```python
from build123d import *

# Parameters (mm, degrees)
SKETCH1_W                    = 40
SKETCH1_H                    = 55
BOSS_EXTRUDE1_DEPTH          = 2
CONVERT_SOLID1_START         = -20
CONVERT_SOLID1_OUTLINE_W     = 55
CONVERT_SOLID1_OUTLINE_H     = 1
CONVERT_SOLID1_DEPTH         = 40
EDGE_FLANGE1_STRIP_W         = 18
EDGE_FLANGE1_STRIP_H         = 3
EDGE_FLANGE1_STRIP_CUT_DEPTH = 40
EDGE_FLANGE1_DEPTH           = 40
SKETCH10_R                   = 2.25
CUT_EXTRUDE1_DEPTH           = 58.965506985


# Read off the part's stored shape, not the designer's step: Convert-Solid1
# Sheet-metal steps are written as plain solids
with BuildPart() as part:
    # Sketch1 → Boss-Extrude1 (new body)
    with BuildSketch(Plane.XY):
        Rectangle(SKETCH1_W, SKETCH1_H)
    extrude(amount=BOSS_EXTRUDE1_DEPTH)

    # Convert-Solid1 outline → Convert-Solid1 (add)
    with BuildSketch(Plane.YZ.offset(CONVERT_SOLID1_START)):
        with Locations((0, -0.5)):
            Rectangle(CONVERT_SOLID1_OUTLINE_W, CONVERT_SOLID1_OUTLINE_H)
    extrude(amount=CONVERT_SOLID1_DEPTH)

    # Edge-Flange1 strip (across the edge) → Edge-Flange1 strip cut (cut)
    with BuildSketch(Plane(origin=(-20, 27.5, -1), x_dir=(0, -1, 0), z_dir=(1, 0, 0))):
        with Locations((-3, -1.5)):
            Rectangle(EDGE_FLANGE1_STRIP_W, EDGE_FLANGE1_STRIP_H)
    extrude(amount=EDGE_FLANGE1_STRIP_CUT_DEPTH, mode=Mode.SUBTRACT)

    # Edge-Flange1 section (across the edge) → Edge-Flange1 (add)
    with BuildSketch(Plane(origin=(-20, 27.5, -1), x_dir=(0, -1, 0), z_dir=(1, 0, 0))):
        with BuildLine():
            Line((0, 3), (0, 15))
            Line((0, 15), (3, 15))
            Line((3, 15), (3, 3))
            ThreePointArc((3, 3), (3.878679656, 0.878679656), (6, 0))
            Line((6, 0), (6, -3))
            ThreePointArc((6, -3), (1.757359313, -1.242640687), (0, 3))
        make_face()
    extrude(amount=EDGE_FLANGE1_DEPTH)

    # Sketch10 → Cut-Extrude1 (cut, through all)
    with BuildSketch(Plane.XZ.offset(-24.5)):
        with Locations(Location((-15, -9, 0), (0, 0, 270))):
            Circle(SKETCH10_R)
        with Locations(Location((0, -9, 0), (0, 0, 270))):
            Circle(SKETCH10_R)
    extrude(amount=-CUT_EXTRUDE1_DEPTH, mode=Mode.SUBTRACT)


solid = part.part
```
Could you check a few things on this model? Use its own coordinates, in mm. A direction names the side the tool comes from. Give positions to 0.01 mm unless a question says otherwise; leave off trailing zeros. Loops run counter-clockwise (first coordinate to the right, second up) from the corner with the lowest first, then second, coordinate; pieces in that order, holes last. Notation, with made-up numbers: (-24.5, 66.5) - (-6.5, 66.5) arc R32 cw to (-6.5, 105.5) - close; hole circle Ø9 at (-9.5, 49.25). An arc over 180 degrees is marked (long way). Use one line per item in the form item = value.
1. I want a section at D-D (y = 23). Please give me the cut outline in (x, z), and give its area (3 significant figures).
Response values:
outline = (-20, -1.4) - (20, -1.4) - (20, 1.81) - (-20, 1.81) - close
area = 128 mm²
2. I want a section at C-C (x = 5). Please give me the cut outline in (y, z).
Response values:
outline = (-27.5, -1) - (21.5, -1) arc R3 cw to (24.5, -4) - (24.5, -16) - (27.5, -16) - (27.5, -4) arc R6 ccw to (21.5, 2) - (-27.5, 2) - close
3. I need wall thicknesses on probe 1 along X at (y, z) = (25.5, -9); probe 2 along Z at (x, y) = (17, 20); probe 3 along Y at (x, z) = (-3, -10). Which ranges of each line are inside material? Lowest first, please.
Response values:
probe_1 = -20 to -17.25, -12.75 to -2.25, 2.25 to 20
probe_2 = -1 to 2
probe_3 = 24.5 to 27.5
4. I'm going to push flat-ended pins straight in: pin 1 Ø2 at (x, z) = (1.5, -6) entering from -Y; pin 2 Ø4 at (x, y) = (-15, -1.5) entering from -Z. Where does each tip first touch, or does it pass through?
Response values:
pin_1 = 24.5
pin_2 = -1
5. On a 3-axis mill with a long thin cutter (end or side, diameter ignored), from which of +Z, -Z, +X, -X, +Y, -Y can I reach the whole of each face in a straight line? I mean faces 1 (the face through (-0.3, 24.5, -11.4)), 2 (the face through (0, 27.5, -13)). Say none if no direction works.
Response values:
face_1 = -Z, +X, -X, -Y
face_2 = +Z, -Z, +X, -X, +Y
6. Thinking about a two-plate mould opening in X: for faces 3 (the face through (0, -3, 2)), 4 (the face through (-20, 4, 0)), 5 (the face through (-16.369, 25.979, -7.214)), which applies, released by +X, released by -X, zero draft, split by the parting line, or undercut?
Response values:
face_3 = zero draft
face_4 = released by -X
face_5 = undercut
7. I want a section at B-B (x = 0). Please give me the cut outline in (y, z).
Response values:
outline = (-27.5, -1) - (21.5, -1) arc R3 cw to (24.5, -4) - (24.5, -6.75) - (27.5, -6.75) - (27.5, -4) arc R6 ccw to (21.5, 2) - (-27.5, 2) - close; (24.5, -16) - (27.5, -16) - (27.5, -11.25) - (24.5, -11.25) - close
8. I want a section at A-A (z = -9). Please give me the cut outline in (x, y).
Response values:
outline = (-20, 24.5) - (-17.25, 24.5) - (-17.25, 27.5) - (-20, 27.5) - close; (-12.75, 24.5) - (-2.25, 24.5) - (-2.25, 27.5) - (-12.75, 27.5) - close; (2.25, 24.5) - (20, 24.5) - (20, 27.5) - (2.25, 27.5) - close
